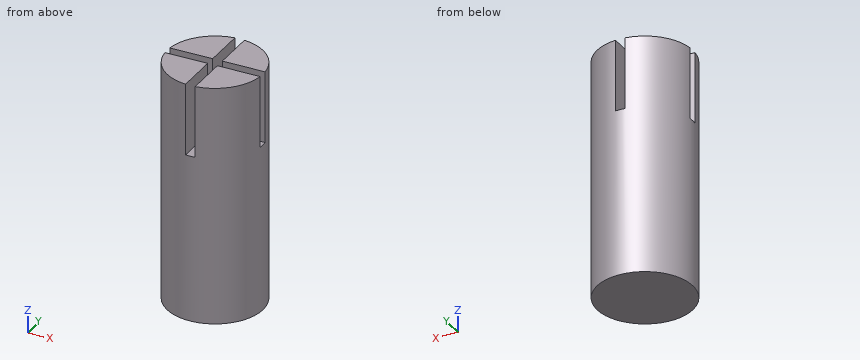
```python
from build123d import *

# Parameters (mm, degrees)
F0_R     = 12.7
F1_DEPTH = 63.5
F2_W     = 2.54
F2_H     = 11.43
F2_H_2   = 2.54
F2_W_2   = 11.43
F3_DEPTH = 19.05


with BuildPart() as f1:
    # F0 (on Top) → F1 (new body)
    with BuildSketch(Plane.XY):
        Circle(F0_R)
    extrude(amount=F1_DEPTH)

    # F2 (on face) → F3 (cut)
    with BuildSketch(Plane.XY.offset(63.5)):
        with Locations((0, 6.985)):
            Rectangle(F2_W, F2_H)
        Rectangle(F2_W, F2_H_2)
        with Locations((-6.985, 0)):
            Rectangle(F2_W_2, F2_H_2)
        with Locations((6.985, 0)):
            Rectangle(F2_W_2, F2_H_2)
        with Locations((0, -6.985)):
            Rectangle(F2_W, F2_H)
    extrude(amount=-F3_DEPTH, mode=Mode.SUBTRACT)


solid = f1.part
```
Verification items for the finished model (mm, model axes). Coordinates: 2 decimals unless noted, no trailing zeros. Order: outer loops, then holes, each group sorted by start corner. A loop starts at its lowest first (then second) coordinate and runs counter-clockwise, first axis right, second up. Notation, with made-up numbers: (85.25, 36.5) -> (132.25, 36.5) arc R16 ccw to (132.25, 65.5) -> close; hole circle Ø1 at (18, 15). An arc over 180 degrees is marked (long way). Answer as CSV lines item,"result". Start each with the question number.
1) Cross-section at D-D, the plane x = 0. Record the boundary of the cut face in (y, z).
2) Material ranges on L1, parallel to X at y = -8.25, z = 47.5; L2, parallel to Y at x = -11, z = 57.5; L3, parallel to Y at x = -0.5, z = 10, recorded low to high. Write a range as [from, to].
3) Cross-section at A-A, the plane z = 58. Record the boundary of the cut face in (x, y), then the cut area to 3 significant figures.
4) Gauge pin test, flat ends, axial feed: pin 1 Ø3.5 at (x, z) = (-9.5, 50.5) entering from -Y; pin 2 Ø8 at (x, z) = (3.5, 24.5) entering from -Y; pin 3 Ø5.5 at (x, z) = (-8, 54.5) entering from +Y; pin 4 Ø12.5 at (x, z) = (4.5, 52.5) entering from -Y. Record the tip position at first contact, or that the pin passes through.
5) Cross-section at C-C, the plane y = 2.25. Record the boundary of the cut face in (x, z), then the cut area to 3 significant figures.
6) Cross-section at B-B, the plane x = -8. Record the boundary of the cut face in (y, z).
Conclusion:
1,outline,"(-12.7, 0) -> (12.7, 0) -> (12.7, 44.45) -> (-12.7, 44.45) -> close"
2,L1,"x = [-9.66, -1.27], [1.27, 9.66]"
2,L2,"y = [-6.35, -1.27], [1.27, 6.35]"
2,L3,"y = [-12.69, 12.69]"
3,outline,"(-12.64, -1.27) arc R12.7 ccw to (-1.27, -12.64) -> (-1.27, -1.27) -> close; (-12.64, 1.27) -> (-1.27, 1.27) -> (-1.27, 12.64) arc R12.7 ccw to start; (1.27, -12.64) arc R12.7 ccw to (12.64, -1.27) -> (1.27, -1.27) -> close; (1.27, 1.27) -> (12.64, 1.27) arc R12.7 ccw to (1.27, 12.64) -> close"
3,area,"384 mm²"
4,pin 1,"stops at y = -10.06"
4,pin 2,"stops at y = -12.7"
4,pin 3,"stops at y = 11.56"
4,pin 4,"stops at y = -12.64"
5,outline,"(-12.5, 0) -> (12.5, 0) -> (12.5, 63.5) -> (1.27, 63.5) -> (1.27, 44.45) -> (-1.27, 44.45) -> (-1.27, 63.5) -> (-12.5, 63.5) -> close"
5,area,"1,540 mm²"
6,outline,"(-9.86, 0) -> (9.86, 0) -> (9.86, 63.5) -> (1.27, 63.5) -> (1.27, 44.45) -> (-1.27, 44.45) -> (-1.27, 63.5) -> (-9.86, 63.5) -> close"
